Geometry check sheet. Reference: the model listing, model coordinates, mm. Face numbers are marked on the shaded views. A direction names the side the tool comes from. Coordinates: 2 decimals unless noted, no trailing zeros. Write each loop counter-clockwise with the first axis right and the second up, starting at its lowest first coordinate (ties: lowest second). Pieces come first, ordered by that corner, then holes. Notation, with made-up numbers: (-4, -17.75) -> (26, -17.75) arc R10 ccw to (26, -0.75) -> close; hole circle Ø10 at (5, -1.5). An arc over 180 degrees is marked (long way). Use a Markdown table: item, result.
Autodesk Inventor part; units mm, degrees
ref_plane "YZ Plane" through (0, 0, 0) normal (1, 0, 0) x (0, 1, 0)
ref_plane "XZ Plane" through (0, 0, 0) normal (0, 1, 0) x (-1, 0, 0)
ref_plane "XY Plane" through (0, 0, 0) normal (0, 0, 1) x (1, 0, 0)
sketch "Sketch1" plane through (0, 0, 0) normal (0, 0, 1) x (1, 0, 0)
  line L0 (-87.8501, 55.3459) -> (-87.8501, 29.9459)
  line L1 (-87.8501, 29.9459) -> (-93.4, 29.9459)
  line L2 (-59.2667, 42.6459) -> (-60.6149, 42.6459)
  line L3 (-59.2667, 42.6459) -> (0, 42.6459) construction
  line L4 (-41.4694, -37.9453) -> (-35.1194, -37.9453)
  line L5 (-93.4, 29.9459) -> (-93.4, 17.2459)
  line L6 (-93.4, 17.2459) -> (-80.7, 17.2459)
  line L7 (-80.7, 17.2459) -> (-74.35, 17.2459)
  line L8 (-74.35, 17.2459) -> (-74.35, -160.6575)
  line L9 (-93.4, 17.2459) -> (-93.4, 7.7209)
  line L10 (-93.4, 17.2459) -> (-83.875, 17.2459) construction
  line L11 (-93.4, 7.7209) -> (-80.7, 7.7209)
  line L12 (-80.7, 7.7209) -> (-80.7, -43.0791)
  line L13 (-80.7, -43.0791) -> (-93.4, -43.0791)
  line L14 (-93.4, 7.7209) -> (-87.05, 7.7209)
  line L15 (-87.05, 7.7209) -> (-87.05, 1.7773)
  line L16 (-87.05, 1.7773) -> (-93.4, 1.7773)
  line L17 (-93.4, 29.9459) -> (-93.4, 7.7209)
  line L18 (-93.4, 1.7773) -> (-93.4, -43.0791)
  line L19 (-80.7, -43.0791) -> (-21.9625, -43.0791) construction
  line L20 (-68, -160.6575) -> (-74.35, -160.6575)
  line L21 (-64.6621, -148.2003) -> (-40.1276, -148.2003) construction
  line L22 (0, 42.6459) -> (0, 0)
  line L23 (-87.8501, 55.3459) -> (-18.3062, 55.3459) construction
  line L24 (-87.8501, 55.3459) -> (-14.7047, 55.3459) construction
  line L25 (-87.8501, 55.3459) -> (-55.5582, 40.2879)
  line L26 (-87.8501, 55.3459) -> (-52.22, 55.3459) construction
  line L27 (-59.2667, 42.6459) -> (-59.2667, -37.9453)
  line L28 (-59.2667, 42.6459) -> (21.3245, 42.6459) construction
  line L29 (-59.2667, -37.9453) -> (-41.4694, -37.9453)
  line L30 (-68, -160.6575) -> (-35.1194, -37.9453)
  dimension "d87" = 25.4
  dimension "d88" = 5.5499
  dimension "d89" = 87.8501
  dimension "d90" = 12.7
  dimension "d92" = 59.2667
  dimension "d93" = 6.35
  dimension "d95" = 12.7
  dimension "d96" = 12.7
  dimension "d97" = 6.35
  dimension "d98" = 9.525
  dimension "d99" = 50.8
  dimension "d100" = 12.7
  dimension "d101" = 6.35
  dimension "d102" = 5.9436
  dimension "d113" = 25
  dimension "d115" = 32.2919
  dimension "d117" = 80.5912
revolve "Revolution2" add sketch "Sketch1" angle 360 about axis through (0, 42.6459, 0) along (0, -1, 0) contours L25 L27 L29 L4 L30 L20 L8 L7 L6 L5 L1 L0 | L2 L27 L25
properties part number "Phenolic 8-inch v1" material "Phenolic Resin"
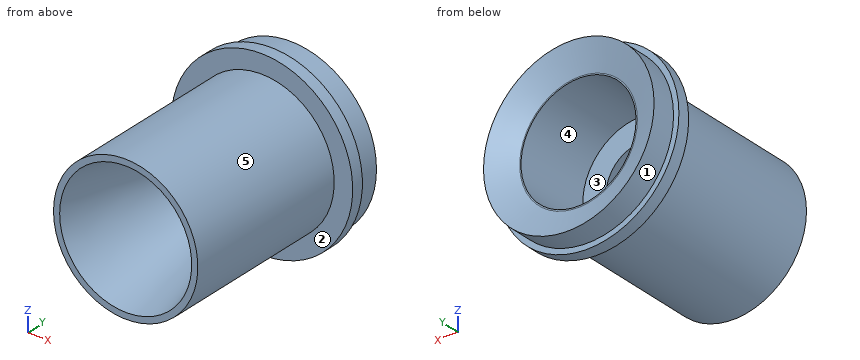
Item 1: Tool access check on the marked faces 4 and 5. Record the directions out of +Z, -Z, +X, -X, +Y, -Y that give a thin tool (end or side, any length) a straight path to the whole face; none if there is none.
Answer block:
| item | result |
|---|---|
| face 4 | +Y |
| face 5 | -Y |
Item 2: Section check A-A on z = 0. Record the boundary of the cut face in (x, y), then the cut area to 3 significant figures.
Answer block:
| item | result |
|---|---|
| outline | (-93.4, 17.25) -> (-74.35, 17.25) -> (-74.35, -160.66) -> (-68, -160.66) -> (-35.12, -37.95) -> (-59.27, -37.95) -> (-59.27, 42.65) -> (-60.61, 42.65) -> (-87.85, 55.35) -> (-87.85, 29.95) -> (-93.4, 29.95) -> close; (35.12, -37.95) -> (68, -160.66) -> (74.35, -160.66) -> (74.35, 17.25) -> (93.4, 17.25) -> (93.4, 29.95) -> (87.85, 29.95) -> (87.85, 55.35) -> (60.61, 42.65) -> (59.27, 42.65) -> (59.27, -37.95) -> close |
| area | 9,200 mm^2 |
Item 3: Section check D-D on y = -53.5. Record the boundary of the cut face in (x, z).
Answer block:
| item | result |
|---|---|
| outline | circle Ø148.7 at (0, 0); hole circle Ø78.57 at (0, 0) |
Item 4: Section check B-B on x = 0. Record the boundary of the cut face in (y, z).
Answer block:
| item | result |
|---|---|
| outline | (-160.66, -74.35) -> (17.25, -74.35) -> (17.25, -93.4) -> (29.95, -93.4) -> (29.95, -87.85) -> (55.35, -87.85) -> (42.65, -60.61) -> (42.65, -59.27) -> (-37.95, -59.27) -> (-37.95, -35.12) -> (-160.66, -68) -> close; (-160.66, 68) -> (-37.95, 35.12) -> (-37.95, 59.27) -> (42.65, 59.27) -> (42.65, 60.61) -> (55.35, 87.85) -> (29.95, 87.85) -> (29.95, 93.4) -> (17.25, 93.4) -> (17.25, 74.35) -> (-160.66, 74.35) -> close |
Item 5: Mould release check, pull along Z, two halves, no side actions. Record for the marked faces 1, 2 and 3: +Z half, -Z half, draft (parallel to the pull), parting line (faces both ways), or undercut.
Answer block:
| item | result |
|---|---|
| face 1 | parting line |
| face 2 | draft |
| face 3 | undercut |
Item 6: Thickness scan on L1, parallel to Z at x = 0, y = 21; L2, parallel to X at y = -9, z = 0. Record the ranges inside material, lowest first. Write a range as [from, to].
Answer block:
| item | result |
|---|---|
| L1 | z = [-93.4, -59.27], [59.27, 93.4] |
| L2 | x = [-74.35, -59.27], [59.27, 74.35] |
Item 7: Depth check by flat-ended pin: P1, Ø1.5, axis at x = -8.5, y = -89, coming from the -Z side (3 decimals); P2, Ø5, axis at y = -38, z = -40.5, coming from the -X side; P3, Ø8, axis at y = -86.5, z = -7.5, coming from the -X side. Enter the tip coordinate at first touch or a pass-through.
Answer block:
| item | result |
|---|---|
| P1 | stops at z = -73.945 |
| P2 | stops at x = -63.91 |
| P3 | stops at x = -74.27 |
Item 8: Section check C-C on y = -7. Record the boundary of the cut face in (x, z).
Answer block:
| item | result |
|---|---|
| outline | circle Ø148.7 at (0, 0); hole circle Ø118.53 at (0, 0) |
